from build123d import *

# Parameters (mm, degrees)
EXTRUDE_THIN1_DEPTH = 7.62


with BuildPart() as part:
    # Sketch1 → Extrude-Thin1 (new, symmetric)
    with BuildSketch(Plane.ZY.offset(-110.25)):
        with BuildLine():
            Line((-615.614704462, 170.984199418), (-802.597206958, 133.923548514))
            ThreePointArc((-802.597206958, 133.923548514), (-908.053927045, 228.674152785), (-787.513709868, 303.298899781))
            Line((-787.513709868, 303.298899781), (-610.022461239, 233.780522747))
            ThreePointArc((-610.022461239, 233.780522747), (-589.286960141, 200.286783656), (-615.614704462, 170.984199418))
        make_face()
        with BuildLine():
            Line((-617.590029198, 180.950326659), (-804.572531695, 143.889675755))
            ThreePointArc((-804.572531695, 143.889675755), (-897.933976221, 227.772933997), (-791.21902444, 293.838654333))
            Line((-791.21902444, 293.838654333), (-613.72777581, 224.320277299))
            ThreePointArc((-613.72777581, 224.320277299), (-599.406910966, 201.188002445), (-617.590029198, 180.950326659))
        make_face(mode=Mode.SUBTRACT)
    extrude(amount=EXTRUDE_THIN1_DEPTH, both=True)


solid = part.part
For this review, take the finished solid that the model builds, in its own axes (mm). A direction names the side the tool comes from. Give positions to 0.01 mm unless a question says otherwise; leave off trailing zeros. Order: outer loops, then holes, each group sorted by start corner. A loop starts at its lowest first (then second) coordinate and runs counter-clockwise, first axis right, second up. Notation, with made-up numbers: M 10,12 L 50,12 A29 ccw 50,51 Z; hole C -28.5,33 d5. An arc over 180 degrees is marked long. Answer in a Markdown table with one row per item. Add a question column.
(1) For faces 1 (the face through (117.87, 274, -736)), 2 (the face through (110.143, 259.566, -703.716)), list the 3-axis set-ups (+Z, -Z, +X, -X, +Y, -Y) from which the entire face can be reached by the end or side of a thin tool; tool diameter is ignored.
(2) Consider section B-B on x = 109.25. State the section outline as (y, z) points (1 decimal).
(3) Consider section A-A on z = -661.5. State the section outline as (x, y) points, and give its area (3 significant figures).
(4) Mouldability with a two-part tool opening along Y and no side actions: class faces 3 (the face through (110.143, 269.026, -700.011)), 4 (the face through (110.143, 201.595, -599.374)), 5 (the face through (102.63, 274, -736)) as +Y half, -Y half, draft (parallel to the pull), parting line (faces both ways), or undercut.
(5) For pin 1 (8 mm diameter, centred on y = 278, z = -862, fed in from +X); pin 2 (6 mm diameter, centred on x = 107.5, y = 185, fed in from +Z); pin 3 (2 mm diameter, centred on x = 116, z = -708.5, fed in from -Y); pin 4 (6 mm diameter, centred on x = 111, y = 191, fed in from +Z), all flat-tipped, find the tip position at first contact; note any pin that passes through.
(6) Consider section C-C on y = 275.5. State the section outline as (x, z) points.
(7) Wall thickness on probe 1 along Y at (x, z) = (106.25, -849); probe 2 along Z at (x, y) = (113, 216); probe 3 along Y at (x, z) = (111.75, -683): over which ranges is each line inside the solid? List them lowest first. Write a range as [from, to].
Evaluation:
| question | item | result |
|---|---|---|
| 1 | face 1 | +Z, -Z, +X, +Y, -Y |
| 1 | face 2 | +X, -X |
| 2 | outline | M 133.9,-802.6 A88.6 ccw long 303.3,-787.5 L 233.8,-610 A32.8 ccw 171,-615.6 Z; hole M 143.9,-804.6 A78.4 ccw long 293.8,-791.2 L 224.3,-613.7 A22.7 ccw 181,-617.6 Z |
| 3 | outline | M 102.63,161.89 L 117.87,161.89 L 117.87,172.25 L 102.63,172.25 Z; M 102.63,243.03 L 117.87,243.03 L 117.87,253.94 L 102.63,253.94 Z |
| 3 | area | 324 mm^2 |
| 4 | face 3 | +Y half |
| 4 | face 4 | undercut |
| 4 | face 5 | draft |
| 5 | pin 1 | passes through |
| 5 | pin 2 | stops at z = -592.89 |
| 5 | pin 3 | stops at y = 152.38 |
| 5 | pin 4 | stops at z = -590.47 |
| 6 | outline | M 102.63,-889.51 L 117.87,-889.51 L 117.87,-876.03 L 102.63,-876.03 Z; M 102.63,-744.4 L 117.87,-744.4 L 117.87,-716.54 L 102.63,-716.54 Z |
| 7 | probe 1 | y = [137.18, 148.02], [293.61, 304.46] |
| 7 | probe 2 | z = [-908.27, -898.1], [-603.27, -591.75] |
| 7 | probe 3 | y = [157.63, 167.99], [251.45, 262.36] |
